Here's how the part is built. I have some questions about the finished solid (model axes, mm). A direction names the side the tool comes from. Round coordinates to 2 decimals unless told otherwise and drop trailing zeros. Order: outer loops, then holes, each group sorted by start corner. A loop starts at its lowest first (then second) coordinate and runs counter-clockwise, first axis right, second up. Notation, with made-up numbers: (33, -9.5) -> (53, -9.5) arc R20 cw to (53, 12.5) -> close; hole circle Ø10 at (-38, 49.5). An arc over 180 degrees is marked (long way). One line per item, written item: value.
```python
from build123d import *

# Parameters (mm, degrees)
BOX323_W          = 10
BOX323_H          = 2.5
BOX323_DEPTH      = 10
CYLINDER152_R     = 1.6
CYLINDER152_DEPTH = 9
CYLINDER153_R     = 1.6
CYLINDER153_DEPTH = 9
CYLINDER154_R     = 1.6
CYLINDER154_DEPTH = 9
CYLINDER155_R     = 1.6
CYLINDER155_DEPTH = 9
BOX071_W          = 30
BOX071_H          = 9
BOX071_DEPTH      = 10
FILLET034_R       = 3


with BuildPart() as cube394:
    # Box323 → Box323 (new body)
    with BuildSketch(Plane(origin=(429.5, -12.5, 5), x_dir=(1, 0, 0), z_dir=(0, 0, 1))):
        with Locations((5, 1.25)):
            Rectangle(BOX323_W, BOX323_H)
    extrude(amount=BOX323_DEPTH)


with BuildPart() as cylinder152:
    # Cylinder152 → Cylinder152 (new body)
    with BuildSketch(Plane(origin=(555, -5, 10), x_dir=(1, 0, 0), z_dir=(0, -1, 0))):
        Circle(CYLINDER152_R)
    extrude(amount=CYLINDER152_DEPTH)


with BuildPart() as fusion125:
    # Cylinder153 → Cylinder153 (new body)
    with BuildSketch(Plane(origin=(450, -5, 10), x_dir=(1, 0, 0), z_dir=(0, -1, 0))):
        Circle(CYLINDER153_R)
    extrude(amount=CYLINDER153_DEPTH)

    # Fusion125: union Cylinder152
    add(cylinder152.part)


with BuildPart() as fusion125_1:
    # Fusion125 placement: moved
    add(fusion125.part.moved(Location((-9, 5, 0))))


with BuildPart() as cylinder154:
    # Cylinder154 → Cylinder154 (new body)
    with BuildSketch(Plane(origin=(555, -5, 10), x_dir=(1, 0, 0), z_dir=(0, -1, 0))):
        Circle(CYLINDER154_R)
    extrude(amount=CYLINDER154_DEPTH)


with BuildPart() as fusion135:
    # Cylinder155 → Cylinder155 (new body)
    with BuildSketch(Plane(origin=(450, -5, 10), x_dir=(1, 0, 0), z_dir=(0, -1, 0))):
        Circle(CYLINDER155_R)
    extrude(amount=CYLINDER155_DEPTH)

    # Fusion132: union Cylinder154
    add(cylinder154.part)


with BuildPart() as fusion135_1:
    # Fusion132 placement: moved
    add(fusion135.part.moved(Location((9, 5, 0))))

    # Fusion135: union Fusion125
    add(fusion125_1.part)


with BuildPart() as fender_spacer_front_left:
    # Box071 → Box071 (new body)
    with BuildSketch(Plane(origin=(435, -9, 5), x_dir=(1, 0, 0), z_dir=(0, 0, 1))):
        with Locations((15, 4.5)):
            Rectangle(BOX071_W, BOX071_H)
    extrude(amount=BOX071_DEPTH)

    # Fillet034
    fillet034_edges = [fender_spacer_front_left.edges().sort_by_distance(p)[0] for p in [
        (435, -4.5, 15),
        (435, -4.5, 5),
        (465, -4.5, 15),
        (465, -4.5, 5),
    ]]
    fillet(fillet034_edges, radius=FILLET034_R)

    # Cut083: cut Fusion135
    add(fusion135_1.part, mode=Mode.SUBTRACT)


with BuildPart() as fender_spacer_front_left_1:
    # Cut083 placement: moved
    add(fender_spacer_front_left.part.moved(Location((0, -10, 0))))

    # Cut322: cut Cube394
    add(cube394.part, mode=Mode.SUBTRACT)


solid = fender_spacer_front_left_1.part
```
Q1. I want a section at A-A on x = 441. Write out the boundary of the cut face in (y, z), then the cut area to 3 significant figures.
Answers:
outline: (-19, 5) -> (-10, 5) -> (-10, 8.4) -> (-19, 8.4) -> close; (-19, 11.6) -> (-10, 11.6) -> (-10, 15) -> (-19, 15) -> close
area: 61.2 mm2
Q2. If we mould it in two halves opening along X, with no side actions, what happens to faces 3 (the face through (465, -15, 10)), 4 (the face through (435.86, -15.7, 14.1)), 5 (the face through (450, -19, 10)), 6 (the face through (442.48, -14.44, 9.39))? For each: pulls with the +X half, pulls with the -X half, needs draft (parallel to the pull), parting line crosses it, or undercut.
Answers:
face 3: pulls with the +X half
face 4: pulls with the -X half
face 5: needs draft
face 6: undercut
Q3. I want a section at D-D on z = 7.5. Write out the boundary of the cut face in (x, y).
Answers:
outline: (435.04, -19) -> (464.96, -19) -> (464.96, -10) -> (439.5, -10) -> (439.5, -12.5) -> (435.04, -12.5) -> close
Q4. I want a section at C-C on z = 10. Write out the boundary of the cut face in (x, y).
Answers:
outline: (435, -19) -> (439.4, -19) -> (439.4, -12.5) -> (435, -12.5) -> close; (442.6, -19) -> (457.4, -19) -> (457.4, -10) -> (442.6, -10) -> close; (460.6, -19) -> (465, -19) -> (465, -10) -> (460.6, -10) -> close
Q5. I need wall thicknesses on line 1 along Z through (x, y) = (441, -16.75); line 2 along X through (y, z) = (-14.25, 11); line 3 along X through (y, z) = (-17, 8.75). Which ranges of each line are inside material? Lowest first, please.
Answers:
line 1: 5 to 8.4, 11.6 to 15
line 2: 435 to 439.75, 442.25 to 457.75, 460.25 to 465
line 3: 435 to 440, 442 to 458, 460 to 465
Q6. I want a section at B-B on y = -16. Write out the boundary of the cut face in (x, z).
Answers:
outline: (435, 8) arc R3 ccw to (438, 5) -> (462, 5) arc R3 ccw to (465, 8) -> (465, 12) arc R3 ccw to (462, 15) -> (438, 15) arc R3 ccw to (435, 12) -> close; hole circle Ø3.2 at (441, 10); hole circle Ø3.2 at (459, 10)
Q7. For P1, Ø1.2, axis at y = -10.5, z = 13.5, coming from the -X side; P2, Ø3, axis at y = -12, z = 6.5, coming from the +X side; P3, Ø3, axis at x = 441, z = 10, coming from the +Y side, each with a flat end and sliding along its axis, tell me the tip position at first contact or that it passes through.
Answers:
P1: x = 439.5
P2: x = 465
P3: through
Q8. Which directions (+Z, -Z, +X, -X, +Y, -Y) give clear straight access to the entire face, cutting with the end or side of a thin tool? Please do faces 1 (the face through (452, -10, 10)), 2 (the face through (439.5, -11, 7)).
Answers:
face 1: +Z, -Z, +X, -X, +Y
face 2: +Z, -Z, -X, +Y
